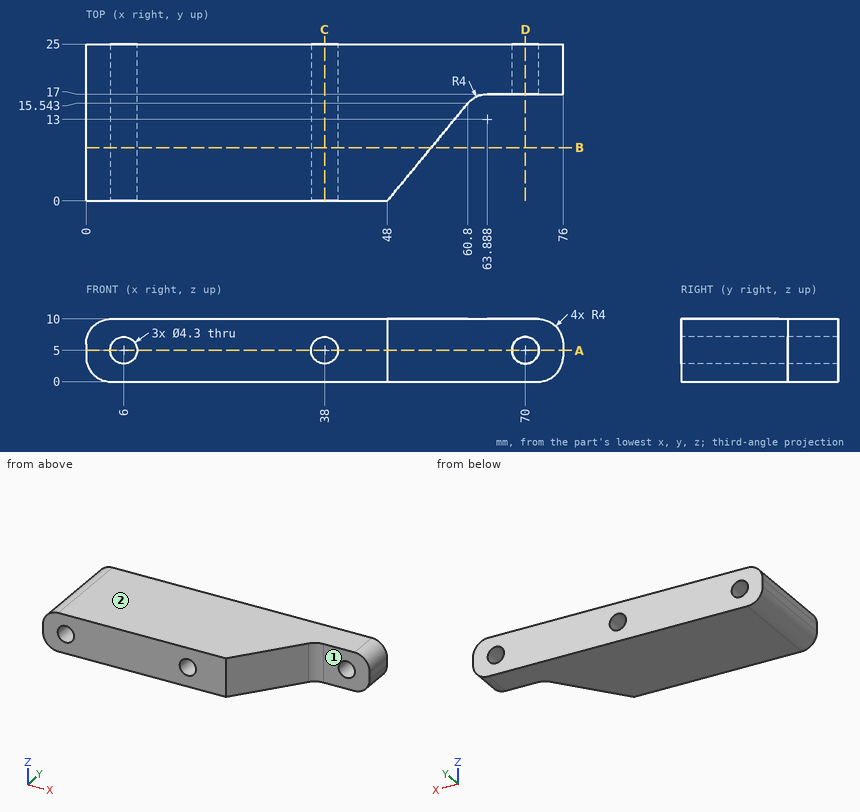
Verification items for this drawing (mm, ordinates from the low corner). A direction names the side the tool comes from. Round coordinates to 2 decimals unless told otherwise and drop trailing zeros. Order: outer loops, then holes, each group sorted by start corner. A loop starts at its lowest first (then second) coordinate and runs counter-clockwise, first axis right, second up. Notation, with made-up numbers: (71, -18.75) - (125, -18.75) arc R26 ccw to (125, 20.25) - close; hole circle Ø9 at (20, 73). An arc over 180 degrees is marked (long way). Use CSV: the item, a comma, the result in double quotes.
(1) Section check B-B on y = 8.5. Record the boundary of the cut face in (x, z).
Entries:
outline,"(0, 4) arc R4 ccw to (4, 0) - (55, 0) - (55, 10) - (4, 10) arc R4 ccw to (0, 6) - close; hole circle Ø4.3 at (6, 5); hole circle Ø4.3 at (38, 5)"
(2) Access from +Z, -Z, +X, -X, +Y, -Y to the whole of each face (thin tool, end or side, straight path). Record for the marked faces 1 and 2.
Entries:
face 1,"+Z, -Z, +X, -Y"
face 2,"+Z, +X, -X, +Y, -Y"
(3) Thickness scan on probe 1 along Z at (x, y) = (6, 11.75); probe 2 along X at (y, z) = (15, 5.25) (1 decimal); probe 3 along Y at (x, z) = (67.5, 1.5). Record the ranges inside material, lowest first. Write a range as from..to.
Entries:
probe 1,"0..2.85, 7.15..10"
probe 2,"0..3.9, 8.1..35.9, 40.1..60.4"
probe 3,"17..25"
(4) Section check A-A on z = 5. Record the boundary of the cut face in (x, y), and give its area (3 significant figures).
Entries:
outline,"(0, 0) - (3.85, 0) - (3.85, 25) - (0, 25) - close; (8.15, 0) - (35.85, 0) - (35.85, 25) - (8.15, 25) - close; (40.15, 0) - (48, 0) - (60.8, 15.54) arc R4 cw to (63.89, 17) - (67.85, 17) - (67.85, 25) - (40.15, 25) - close; (72.15, 17) - (76, 17) - (76, 25) - (72.15, 25) - close"
area,"1,290 mm^2"
(5) Section check D-D on x = 70. Record the boundary of the cut face in (y, z), and give its area (3 significant figures).
Entries:
outline,"(17, 0) - (25, 0) - (25, 2.85) - (17, 2.85) - close; (17, 7.15) - (25, 7.15) - (25, 10) - (17, 10) - close"
area,"45.6 mm^2"
(6) Section check C-C on x = 38. Record the boundary of the cut face in (y, z).
Entries:
outline,"(0, 0) - (25, 0) - (25, 2.85) - (0, 2.85) - close; (0, 7.15) - (25, 7.15) - (25, 10) - (0, 10) - close"
